Input: dimensioned drawing with shaded views. Units: mm. Origin: part minimum x, y, z. Round coordinates to 2 decimals unless told otherwise and drop trailing zeros. Write each loop counter-clockwise with the first axis right and the second up, starting at its lowest first coordinate (ties: lowest second). Pieces come first, ordered by that corner, then holes. Notation, with made-up numbers: (41, -37) - (52, -37) arc R14 cw to (52, -18) - close; hole circle Ø10 at (41.5, 68.25). An arc over 180 degrees is marked (long way). Use one line per item in the form item = value.
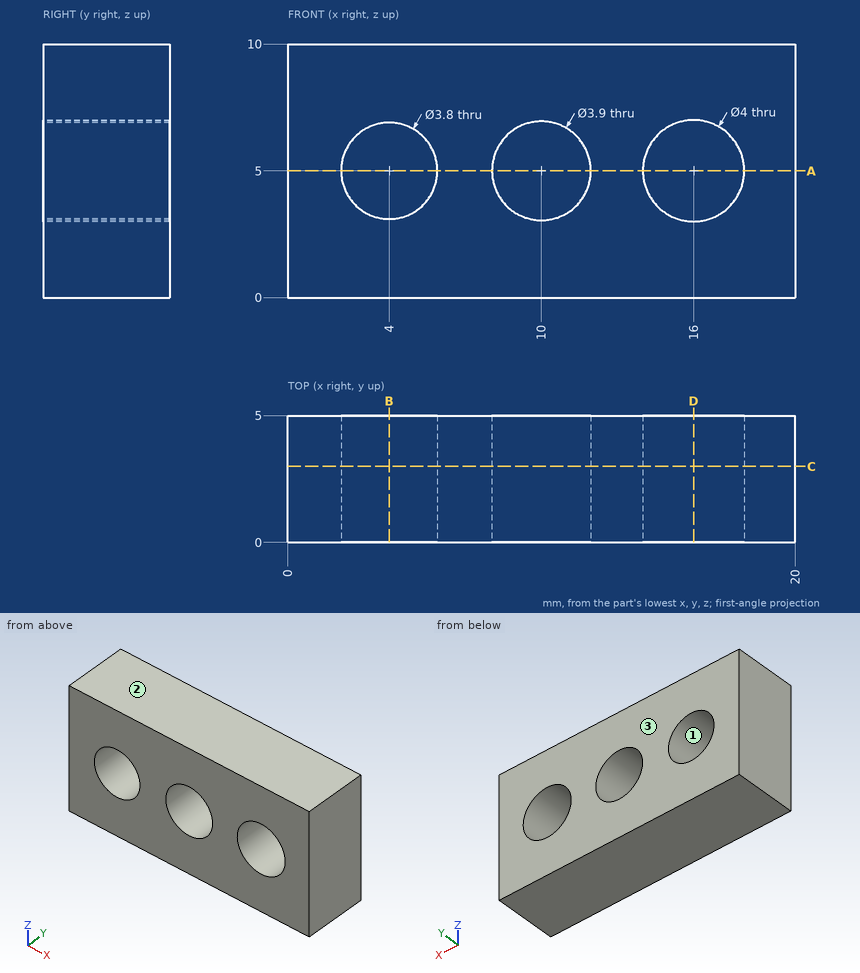
(1) Material intervals for L1, parallel to X at y = 1.25, z = 5; L2, parallel to Z at x = 17, y = 4.7; L3, parallel to Z at x = 16.75, y = 0.55, sorted ascending.
Derived:
L1 = 0 to 2.1, 5.9 to 8.05, 11.95 to 14, 18 to 20
L2 = 0 to 3.27, 6.73 to 10
L3 = 0 to 3.15, 6.85 to 10
(2) First-contact query: pin 1 Ø1.5 at (x, z) = (14, 6) entering from -Y. Flat tip, straight axial feed; report the tip coordinate or a pass-through.
Derived:
pin_1 = 0
(3) Cut plane B-B on x = 4. Output: boundary loops of the cut face in (y, z).
Derived:
outline = (0, 0) - (5, 0) - (5, 3.1) - (0, 3.1) - close; (0, 6.9) - (5, 6.9) - (5, 10) - (0, 10) - close
(4) Cut plane C-C on y = 3. Output: boundary loops of the cut face in (x, z).
Derived:
outline = (0, 0) - (20, 0) - (20, 10) - (0, 10) - close; hole circle Ø3.8 at (4, 5); hole circle Ø3.9 at (10, 5); hole circle Ø4 at (16, 5)
(5) Cut plane A-A on z = 5. Output: boundary loops of the cut face in (x, y), then the cut area to 3 significant figures.
Derived:
outline = (0, 0) - (2.1, 0) - (2.1, 5) - (0, 5) - close; (5.9, 0) - (8.05, 0) - (8.05, 5) - (5.9, 5) - close; (11.95, 0) - (14, 0) - (14, 5) - (11.95, 5) - close; (18, 0) - (20, 0) - (20, 5) - (18, 5) - close
area = 41.5 mm^2
(6) Draft query along Z for the marked faces 1, 2 and 3. Return one class per face: released by +Z, released by -Z, zero draft, split by the parting line, or undercut.
Derived:
face_1 = undercut
face_2 = released by +Z
face_3 = zero draft
(7) Cut plane D-D on x = 16. Output: boundary loops of the cut face in (y, z), then the cut area to 3 significant figures.
Derived:
outline = (0, 0) - (5, 0) - (5, 3) - (0, 3) - close; (0, 7) - (5, 7) - (5, 10) - (0, 10) - close
area = 30.0 mm^2
